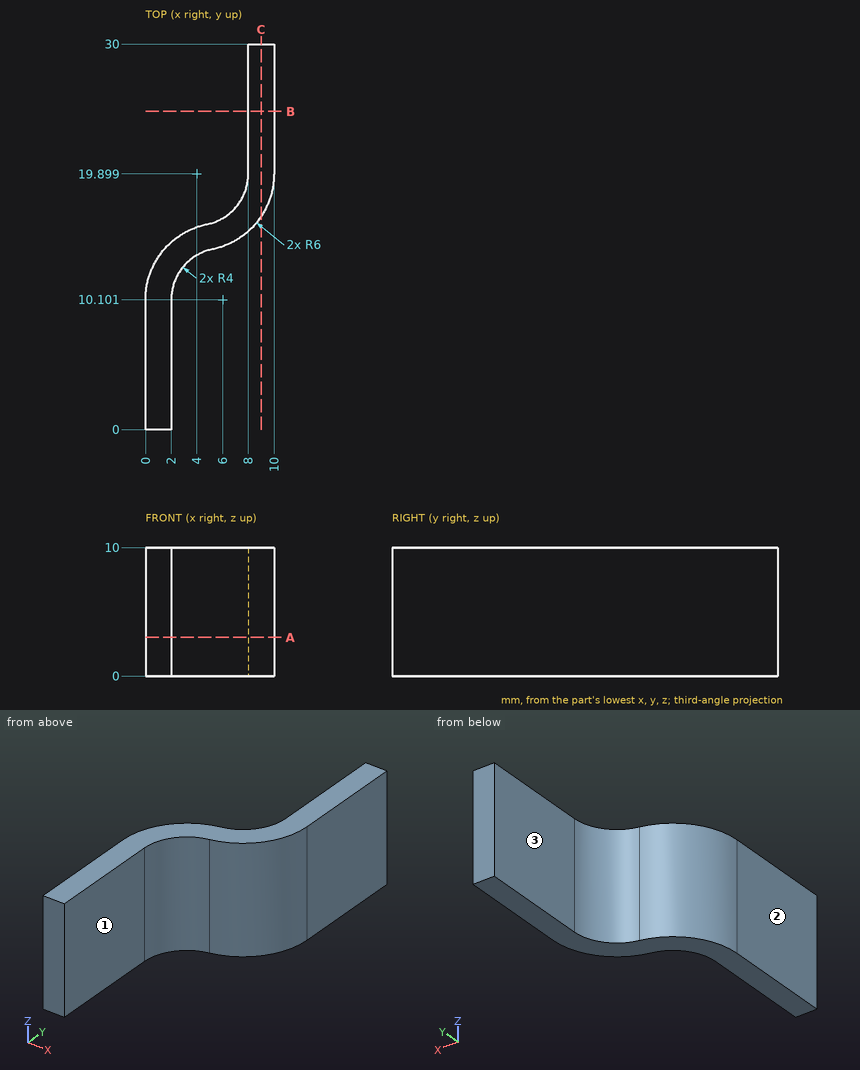
Here's the drawing with two shaded views (mm, measured from the low corner). I have some questions. A direction names the side the tool comes from. Round coordinates to 2 decimals unless told otherwise and drop trailing zeros. Loops run counter-clockwise (first coordinate to the right, second up) from the corner with the lowest first, then second, coordinate; pieces in that order, holes last. Notation, with made-up numbers: (-25.5, 87.5) - (-6.5, 87.5) arc R32 ccw to (-6.5, 117.5) - close; hole circle Ø6 at (5.5, -16). An arc over 180 degrees is marked (long way). Write item = value, one per line.
1) I need wall thicknesses on line 1 along X through (y, z) = (28, 5.75); line 2 along X through (y, z) = (2.75, 6); line 3 along Y through (x, z) = (0.5, 5.75). Which ranges of each line are inside material? Lowest first, please. Write a range as from..to.
Computed:
line_1 = 8..10
line_2 = 0..2
line_3 = 0..12.5
2) I'm going to push flat-ended pins straight in: P1, Ø3, axis at x = 2, z = 1, coming from the +Y side; P2, Ø5, axis at y = 4, z = 7, coming from the +X side; P3, Ø4, axis at y = 17.5, z = 1, coming from the -X side. Where does each tip first touch, or does it pass through?
Computed:
P1 = 15.56
P2 = 2
P3 = 3.38
3) Imagine slicing it at B-B (y = 24.75). Please give me the cut outline in (x, z), and give its area (3 significant figures).
Computed:
outline = (8, 0) - (10, 0) - (10, 10) - (8, 10) - close
area = 20.0 mm2
4) On a 3-axis mill with a long thin cutter (end or side, diameter ignored), from which of +Z, -Z, +X, -X, +Y, -Y can I reach the whole of each face in a straight line? I mean the marked faces 1, 2 and 3. Say none if no direction works.
Computed:
face_1 = +Z, -Z, +X, -Y
face_2 = +Z, -Z, -X, +Y, -Y
face_3 = +Z, -Z, -X, +Y
5) Imagine slicing it at A-A (z = 3). Please give me the cut outline in (x, y), and give its area (3 significant figures).
Computed:
outline = (0, 0) - (2, 0) - (2, 10.1) arc R4 cw to (5.2, 14.02) arc R6 ccw to (10, 19.9) - (10, 30) - (8, 30) - (8, 19.9) arc R4 cw to (4.8, 15.98) arc R6 ccw to (0, 10.1) - close
area = 67.8 mm2
6) Imagine slicing it at C-C (x = 9). Please give me the cut outline in (y, z), and give its area (3 significant figures).
Computed:
outline = (16.58, 0) - (30, 0) - (30, 10) - (16.58, 10) - close
area = 134 mm2
